from build123d import *

# Parameters (mm, degrees)
EXTRUDE_1_DEPTH = 100


with BuildPart() as part:
    # 草图1 → 凸台-拉伸1 (new body)
    with BuildSketch(Plane.XY):
        with BuildLine():
            Line((-17.468782805, -13.940182328), (0.281217195, -13.940182328))
            Line((0.281217195, -13.940182328), (1.031217195, -13.507169626))
            Line((1.031217195, -13.507169626), (1.781217195, -13.940182328))
            Line((1.781217195, -13.940182328), (19.531217195, -13.940182328))
            ThreePointArc((19.531217195, -13.940182328), (20.591877367, -13.5008425), (21.031217195, -12.440182328))
            Line((21.031217195, -12.440182328), (21.031217195, -5.640182328))
            Line((21.031217195, -5.640182328), (17.031217195, -5.640182328))
            Line((17.031217195, -5.640182328), (17.031217195, -8.240182328))
            Line((17.031217195, -8.240182328), (18.131217195, -8.240182328))
            ThreePointArc((18.131217195, -8.240182328), (18.343349229, -8.328050294), (18.431217195, -8.540182328))
            Line((18.431217195, -8.540182328), (18.431217195, -11.040182328))
            ThreePointArc((18.431217195, -11.040182328), (18.343349229, -11.252314363), (18.131217195, -11.340182328))
            Line((18.131217195, -11.340182328), (11.031217195, -11.340182328))
            Line((11.031217195, -11.340182328), (11.031217195, -2.190182328))
            Line((11.031217195, -2.190182328), (10.598204493, -1.440182328))
            Line((10.598204493, -1.440182328), (11.031217195, -0.690182328))
            Line((11.031217195, -0.690182328), (11.031217195, 4.221340041))
            Line((11.031217195, 4.221340041), (17.919085161, 11.109208006))
            ThreePointArc((17.919085161, 11.109208006), (18.246022225, 11.174239832), (18.431217195, 10.897075972))
            Line((18.431217195, 10.897075972), (18.431217195, 5.659817672))
            ThreePointArc((18.431217195, 5.659817672), (18.343349229, 5.447685637), (18.131217195, 5.359817672))
            Line((18.131217195, 5.359817672), (17.031217195, 5.359817672))
            Line((17.031217195, 5.359817672), (17.031217195, 2.759817672))
            Line((17.031217195, 2.759817672), (21.031217195, 2.759817672))
            Line((21.031217195, 2.759817672), (21.031217195, 14.559817672))
            ThreePointArc((21.031217195, 14.559817672), (20.591877367, 15.620477844), (19.531217195, 16.059817672))
            Line((19.531217195, 16.059817672), (5.231217195, 16.059817672))
            Line((5.231217195, 16.059817672), (5.231217195, 12.059817672))
            Line((5.231217195, 12.059817672), (7.831217195, 12.059817672))
            Line((7.831217195, 12.059817672), (7.831217195, 13.459817672))
            Line((7.831217195, 13.459817672), (15.868475495, 13.459817672))
            ThreePointArc((15.868475495, 13.459817672), (16.145639355, 13.274622702), (16.080607529, 12.947685637))
            Line((16.080607529, 12.947685637), (9.192739564, 6.059817672))
            Line((9.192739564, 6.059817672), (-7.130305174, 6.059817672))
            Line((-7.130305174, 6.059817672), (-14.01817314, 12.947685637))
            ThreePointArc((-14.01817314, 12.947685637), (-14.083204965, 13.274622702), (-13.806041105, 13.459817672))
            Line((-13.806041105, 13.459817672), (-5.768782805, 13.459817672))
            Line((-5.768782805, 13.459817672), (-5.768782805, 12.059817672))
            Line((-5.768782805, 12.059817672), (-3.168782805, 12.059817672))
            Line((-3.168782805, 12.059817672), (-3.168782805, 16.059817672))
            Line((-3.168782805, 16.059817672), (-17.468782805, 16.059817672))
            ThreePointArc((-17.468782805, 16.059817672), (-18.529442977, 15.620477844), (-18.968782805, 14.559817672))
            Line((-18.968782805, 14.559817672), (-18.968782805, 2.759817672))
            Line((-18.968782805, 2.759817672), (-14.968782805, 2.759817672))
            Line((-14.968782805, 2.759817672), (-14.968782805, 5.359817672))
            Line((-14.968782805, 5.359817672), (-16.368782805, 5.359817672))
            Line((-16.368782805, 5.359817672), (-16.368782805, 10.897075972))
            ThreePointArc((-16.368782805, 10.897075972), (-16.183587835, 11.174239832), (-15.856650771, 11.109208006))
            Line((-15.856650771, 11.109208006), (-8.968782805, 4.221340041))
            Line((-8.968782805, 4.221340041), (-8.968782805, -0.690182328))
            Line((-8.968782805, -0.690182328), (-8.535770103, -1.440182328))
            Line((-8.535770103, -1.440182328), (-8.968782805, -2.190182328))
            Line((-8.968782805, -2.190182328), (-8.968782805, -11.340182328))
            Line((-8.968782805, -11.340182328), (-16.068782805, -11.340182328))
            ThreePointArc((-16.068782805, -11.340182328), (-16.280914839, -11.252314363), (-16.368782805, -11.040182328))
            Line((-16.368782805, -11.040182328), (-16.368782805, -8.540182328))
            ThreePointArc((-16.368782805, -8.540182328), (-16.280914839, -8.328050294), (-16.068782805, -8.240182328))
            Line((-16.068782805, -8.240182328), (-14.968782805, -8.240182328))
            Line((-14.968782805, -8.240182328), (-14.968782805, -5.640182328))
            Line((-14.968782805, -5.640182328), (-18.968782805, -5.640182328))
            Line((-18.968782805, -5.640182328), (-18.968782805, -12.440182328))
            ThreePointArc((-18.968782805, -12.440182328), (-18.529442977, -13.5008425), (-17.468782805, -13.940182328))
        make_face()
        with BuildLine():
            Line((-6.368782805, 3.459817672), (-2.827539081, 3.459817672))
            ThreePointArc((-2.827539081, 3.459817672), (1.031217195, 4.796804124), (4.889973471, 3.459817672))
            Line((4.889973471, 3.459817672), (8.431217195, 3.459817672))
            Line((8.431217195, 3.459817672), (8.431217195, -0.140182328))
            Line((8.431217195, -0.140182328), (7.131217195, -0.140182328))
            ThreePointArc((7.131217195, -0.140182328), (7.268203647, -1.440182328), (7.131217195, -2.740182328))
            Line((7.131217195, -2.740182328), (8.431217195, -2.740182328))
            Line((8.431217195, -2.740182328), (8.431217195, -11.340182328))
            Line((8.431217195, -11.340182328), (2.331217195, -11.340182328))
            Line((2.331217195, -11.340182328), (2.331217195, -8.840182328))
            ThreePointArc((2.331217195, -8.840182328), (3.622241119, -8.492600001), (4.831217195, -7.921694497))
            Line((4.831217195, -7.921694497), (4.18568736, -6.82063937))
            ThreePointArc((4.18568736, -6.82063937), (1.031217195, -7.67716878), (-2.12325297, -6.82063937))
            Line((-2.12325297, -6.82063937), (-2.768782805, -7.921694497))
            ThreePointArc((-2.768782805, -7.921694497), (-1.559806729, -8.492600001), (-0.268782805, -8.840182328))
            Line((-0.268782805, -8.840182328), (-0.268782805, -11.340182328))
            Line((-0.268782805, -11.340182328), (-6.368782805, -11.340182328))
            Line((-6.368782805, -11.340182328), (-6.368782805, -2.740182328))
            Line((-6.368782805, -2.740182328), (-5.068782805, -2.740182328))
            ThreePointArc((-5.068782805, -2.740182328), (-5.205769257, -1.440182328), (-5.068782805, -0.140182328))
            Line((-5.068782805, -0.140182328), (-6.368782805, -0.140182328))
            Line((-6.368782805, -0.140182328), (-6.368782805, 3.459817672))
        make_face(mode=Mode.SUBTRACT)
    extrude(amount=EXTRUDE_1_DEPTH)


solid = part.part
Verification items for the finished model (mm, model axes). A direction names the side the tool comes from. Round coordinates to 2 decimals unless told otherwise and drop trailing zeros. Loops run counter-clockwise (first coordinate to the right, second up) from the corner with the lowest first, then second, coordinate; pieces in that order, holes last. Notation, with made-up numbers: (11, 42) - (65, 42) arc R10 ccw to (65, 61) - close; hole circle Ø2 at (66.25, -16.5). An arc over 180 degrees is marked (long way). Write item = value, one per line.
Q1. Sectioned sample at C-C on x = 14. Record the boundary of the cut face in (y, z), plus the area to 3 significant figures.
Here are the results:
outline = (-13.94, 0) - (-11.34, 0) - (-11.34, 100) - (-13.94, 100) - close; (7.19, 0) - (10.87, 0) - (10.87, 100) - (7.19, 100) - close; (13.46, 0) - (16.06, 0) - (16.06, 100) - (13.46, 100) - close
area = 888 mm^2
Q2. Tool access check on faces 3 (the flat face through (-8.969, -7, 49)), 4 (the flat face through (12, 16.06, 49)), 5 (the flat face through (-3.169, 14, 49)). Record the directions out of +Z, -Z, +X, -X, +Y, -Y that give a thin tool (end or side, any length) a straight path to the whole face; none if there is none.
Here are the results:
face_3 = +Z, -Z
face_4 = +Z, -Z, +X, -X, +Y
face_5 = +Z, -Z, +Y
Q3. Material ranges on L1, parallel to Y at x = 6, z = 21; L2, parallel to X at y = -11, z = 92.5; L3, parallel to X at y = 3, z = 36, recorded low to high.
Here are the results:
L1 = -13.94 to -11.34, 3.46 to 6.06, 12.06 to 16.06
L2 = -18.97 to -16.37, -8.97 to -6.37, -0.27 to 2.33, 8.43 to 11.03, 18.43 to 21.03
L3 = -18.97 to -14.97, -8.97 to -6.37, 8.43 to 11.03, 17.03 to 21.03
Q4. Sectioned sample at A-A on y = 1.5. Record the boundary of the cut face in (x, z), plus the area to 3 significant figures.
Here are the results:
outline = (-8.97, 0) - (-6.37, 0) - (-6.37, 100) - (-8.97, 100) - close; (8.43, 0) - (11.03, 0) - (11.03, 100) - (8.43, 100) - close
area = 520 mm^2
Q5. Mould release check, pull along X, two halves, no side actions. Record for faces 1 (the flat face through (-9, -13.94, 49)), 2 (the flat face through (-8.969, 2, 49)): +X half, -X half, draft (parallel to the pull), parting line (faces both ways), or undercut.
Here are the results:
face_1 = draft
face_2 = undercut
Q6. Sectioned sample at B-B on y = -10. Record the boundary of the cut face in (x, z).
Here are the results:
outline = (-18.97, 0) - (-16.37, 0) - (-16.37, 100) - (-18.97, 100) - close; (-8.97, 0) - (-6.37, 0) - (-6.37, 100) - (-8.97, 100) - close; (-0.27, 0) - (2.33, 0) - (2.33, 100) - (-0.27, 100) - close; (8.43, 0) - (11.03, 0) - (11.03, 100) - (8.43, 100) - close; (18.43, 0) - (21.03, 0) - (21.03, 100) - (18.43, 100) - close
